from build123d import *

# Parameters (mm, degrees)
SKETCH2_W           = 50
SKETCH2_H           = 25
BOSS_EXTRUDE1_DEPTH = 10
SKETCH3_W           = 5
SKETCH3_H           = 5.034252603
SKETCH3_H_2         = 5
CUT_EXTRUDE1_DEPTH  = 30.685855218
CUT_EXTRUDE2_DEPTH  = 30.685855218


with BuildPart() as part:
    # Sketch2 → Boss-Extrude1 (new body)
    with BuildSketch(Plane(origin=(0, 0, 0), x_dir=(1, 0, 0), z_dir=(0, 1, 0))):
        Rectangle(SKETCH2_W, SKETCH2_H)
    extrude(amount=BOSS_EXTRUDE1_DEPTH)

    # Sketch3 → Cut-Extrude1 (cut, through all)
    with BuildSketch(Plane(origin=(0, 10, 0), x_dir=(1, 0, 0), z_dir=(0, 1, 0))):
        with Locations((22.5, 9.982873699)):
            Rectangle(SKETCH3_W, SKETCH3_H)
        with Locations((22.5, -10)):
            Rectangle(SKETCH3_W, SKETCH3_H_2)
    cut_extrude1 = extrude(amount=-CUT_EXTRUDE1_DEPTH, mode=Mode.SUBTRACT)

    # Mirror1: Cut-Extrude1 across plane
    add(cut_extrude1.mirror(Plane(origin=(0, 0, 0), x_dir=(0, 0, 1), z_dir=(1, 0, 0))), mode=Mode.SUBTRACT)

    # Sketch4 → Cut-Extrude2 (cut, through all)
    with BuildSketch(Plane(origin=(0, 10, 0), x_dir=(1, 0, 0), z_dir=(0, 1, 0))):
        with BuildLine():
            Line((-13.75, 2.5), (13.75, 2.5))
            ThreePointArc((13.75, 2.5), (16.25, 0), (13.75, -2.5))
            Line((13.75, -2.5), (-13.75, -2.5))
            ThreePointArc((-13.75, -2.5), (-16.25, 0), (-13.75, 2.5))
        make_face()
    extrude(amount=-CUT_EXTRUDE2_DEPTH, mode=Mode.SUBTRACT)


solid = part.part
Input: part model. Units: mm. Frame: model coordinates. A direction names the side the tool comes from. Round coordinates to 2 decimals unless told otherwise and drop trailing zeros. Order: outer loops, then holes, each group sorted by start corner. A loop starts at its lowest first (then second) coordinate and runs counter-clockwise, first axis right, second up. Notation, with made-up numbers: (-33.75, 46) - (22.25, 46) arc R30 cw to (22.25, 79) - close; hole circle Ø11 at (-19.5, -38). An arc over 180 degrees is marked (long way). Use a Markdown table: item, result.
1. Access query for faces 1 (the face through (-20, 5, 10)), 2 (the face through (-20, 5, -10)), 3 (the face through (22, 5, 7.5)), 4 (the face through (20, 5, -10)). Directions: +Z, -Z, +X, -X, +Y, -Y. A direction counts if a zero-diameter tool reaches every point of the face in a straight line with its end or side. Return the directions, or none.
Evaluation:
| item | result |
|---|---|
| face 1 | +Z, -X, +Y, -Y |
| face 2 | -Z, -X, +Y, -Y |
| face 3 | +Z, +X, +Y, -Y |
| face 4 | -Z, +X, +Y, -Y |
2. Section A-A on x = -4. Return the cut outline in (y, z).
Evaluation:
| item | result |
|---|---|
| outline | (0, -12.5) - (10, -12.5) - (10, -2.5) - (0, -2.5) - close; (0, 2.5) - (10, 2.5) - (10, 12.5) - (0, 12.5) - close |
3. Mould query, pull axis Z, two halves, no side actions, for faces 5 (the face through (16.25, 5.07, -0.05)), 6 (the face through (0, 0, -3)), 7 (the face through (0, 5, -12.5)). Classes: +Z half, -Z half, draft (parallel to the pull), parting line (faces both ways), or undercut.
Evaluation:
| item | result |
|---|---|
| face 5 | undercut |
| face 6 | draft |
| face 7 | -Z half |
4. First-contact query: pin 1 (4 mm diameter, centred on x = 23.5, y = 4, fed in from -Z); pin 2 (2.5 mm diameter, centred on y = 6.5, z = 9.5, fed in from +X); pin 3 (4 mm diameter, centred on x = -23, y = 3, fed in from +Z). Flat tips, straight axial feed; report the tip coordinate or a pass-through.
Evaluation:
| item | result |
|---|---|
| pin 1 | z = -7.47 |
| pin 2 | x = 20 |
| pin 3 | z = 7.5 |
5. Section C-C on y = 2. Return the cut outline in (x, z), then the cut area to 3 significant figures.
Evaluation:
| item | result |
|---|---|
| outline | (-25, -7.47) - (-20, -7.47) - (-20, -12.5) - (20, -12.5) - (20, -7.47) - (25, -7.47) - (25, 7.5) - (20, 7.5) - (20, 12.5) - (-20, 12.5) - (-20, 7.5) - (-25, 7.5) - close; hole (-13.75, -2.5) - (13.75, -2.5) arc R2.5 ccw to (13.75, 2.5) - (-13.75, 2.5) arc R2.5 ccw to start |
| area | 993 mm^2 |
6. Section D-D on z = 10.25. Return the cut outline in (x, y).
Evaluation:
| item | result |
|---|---|
| outline | (-20, 0) - (20, 0) - (20, 10) - (-20, 10) - close |
7. Section B-B on z = 0. Return the cut outline in (x, y).
Evaluation:
| item | result |
|---|---|
| outline | (-25, 0) - (-16.25, 0) - (-16.25, 10) - (-25, 10) - close; (16.25, 0) - (25, 0) - (25, 10) - (16.25, 10) - close |
8. Material intervals for probe 1 along Z at (x, y) = (5, 7.5); probe 2 along X at (y, z) = (1.25, -9.5); probe 3 along Z at (x, y) = (23.5, 8), sorted ascending.
Evaluation:
| item | result |
|---|---|
| probe 1 | -12.5 to -2.5, 2.5 to 12.5 |
| probe 2 | -20 to 20 |
| probe 3 | -7.47 to 7.5 |
